Geometry: final body of the model. Coordinates: model frame, mm. Coordinates: 2 decimals unless noted, no trailing zeros. Order: outer loops, then holes, each group sorted by start corner. A loop starts at its lowest first (then second) coordinate and runs counter-clockwise, first axis right, second up. Notation, with made-up numbers: (87.25, -19) - (94.25, -19) arc R10 ccw to (94.25, -15) - close; hole circle Ø10 at (51.5, 43). An arc over 180 degrees is marked (long way). Use a Markdown table: item, result. Add a question column.
```python
from build123d import *

# Parameters (mm, degrees)
SKETCH_1_W          = 50
SKETCH_1_H          = 50
EXTRUDE_1_DEPTH     = 10
FILLET_1_R          = 10
SKETCH_2_R          = 5
CUT_EXTRUDE_1_DEPTH = 10
FILLET_2_R          = 3


with BuildPart() as part:
    # 草图1 → 凸台-拉伸1 (new body)
    with BuildSketch(Plane(origin=(0, 0, 0), x_dir=(1, 0, 0), z_dir=(0, 1, 0))):
        Rectangle(SKETCH_1_W, SKETCH_1_H)
    extrude(amount=EXTRUDE_1_DEPTH)

    # 圆角1
    fillet_1_edges = [part.edges().sort_by_distance(p)[0] for p in [
        (25, 5, 25),
        (-25, 5, 25),
        (-25, 5, -25),
        (25, 5, -25),
    ]]
    fillet(fillet_1_edges, radius=FILLET_1_R)

    # 草图2 → 切除-拉伸1 (cut)
    with BuildSketch(Plane(origin=(0, 10, 0), x_dir=(1, 0, 0), z_dir=(0, 1, 0))):
        Circle(SKETCH_2_R)
    extrude(amount=-CUT_EXTRUDE_1_DEPTH, mode=Mode.SUBTRACT)

    # 圆角2
    fillet_2_edges = [part.edges().sort_by_distance(p)[0] for p in [
        (0, 10, 25),
        (-25, 10, 0),
        (25, 10, 0),
        (0, 10, -25),
        (22.071067812, 10, 22.071067812),
        (22.071067812, 10, -22.071067812),
        (-22.071067812, 10, -22.071067812),
        (-22.071067812, 10, 22.071067812),
        (-5, 10, 0),
    ]]
    fillet(fillet_2_edges, radius=FILLET_2_R)


solid = part.part
```
1) Section D-D (y = 8.5). Return loops of the section in (x, z), then the cut area to 3 significant figures.
2) Section C-C (y = 1.5). Return loops of the section in (x, z), then the cut area to 3 significant figures.
3) Pin query (flat end, axial travel): pin 1 (1.5 mm diameter, centred on y = 1, z = -16, fed in from +X). Return the tip coordinate at first contact, or that it passes through.
4) Ray query, line 1 along Z through (x, y) = (0, 3.5); line 2 along X through (y, z) = (1.25, 4.5). Return the intervals inside material, ascending.
5) Section B-B (x = 0). Return loops of the section in (y, z), then the cut area to 3 significant figures.
6) Section A-A (z = 0). Return loops of the section in (x, y).
7) Draft query along Z for faces 1 (the face through (-0.21, 9.14, -24.1)), 2 (the face through (24.1, 9.14, -0.21)), 3 (the face through (0.21, 9.14, 24.1)), 4 (the face through (-1.08, 3.55, 4.88)). Return one class per face: pulls with the +Z half, pulls with the -Z half, needs draft (parallel to the pull), parting line crosses it, or undercut.
Values follow:
| question | item | result |
|---|---|---|
| 1 | outline | (-24.6, -15) arc R9.6 ccw to (-15, -24.6) - (15, -24.6) arc R9.6 ccw to (24.6, -15) - (24.6, 15) arc R9.6 ccw to (15, 24.6) - (-15, 24.6) arc R9.6 ccw to (-24.6, 15) - close; hole circle Ø10.8 at (0, 0) |
| 1 | area | 2,250 mm² |
| 2 | outline | (-25, -15) arc R10 ccw to (-15, -25) - (15, -25) arc R10 ccw to (25, -15) - (25, 15) arc R10 ccw to (15, 25) - (-15, 25) arc R10 ccw to (-25, 15) - close; hole circle Ø10 at (0, 0) |
| 2 | area | 2,340 mm² |
| 3 | pin 1 | stops at x = 25 |
| 4 | line 1 | z = -25 to -5, 5 to 25 |
| 4 | line 2 | x = -25 to -2.18, 2.18 to 25 |
| 5 | outline | (0, -25) - (7, -25) arc R3 ccw to (10, -22) - (10, -8) arc R3 ccw to (7, -5) - (0, -5) - close; (0, 5) - (7, 5) arc R3 ccw to (10, 8) - (10, 22) arc R3 ccw to (7, 25) - (0, 25) - close |
| 5 | area | 392 mm² |
| 6 | outline | (-25, 0) - (-5, 0) - (-5, 7) arc R3 ccw to (-8, 10) - (-22, 10) arc R3 ccw to (-25, 7) - close; (5, 0) - (25, 0) - (25, 7) arc R3 ccw to (22, 10) - (8, 10) arc R3 ccw to (5, 7) - close |
| 7 | face 1 | pulls with the -Z half |
| 7 | face 2 | needs draft |
| 7 | face 3 | pulls with the +Z half |
| 7 | face 4 | undercut |
